```python
from build123d import *

# Parameters (mm, degrees)
SKETCH1_R           = 1.6
BOSS_EXTRUDE1_DEPTH = 9
FILLET1_R           = 10


with BuildPart() as part:
    # Sketch1 → Boss-Extrude1 (new body)
    with BuildSketch(Plane.XY):
        with BuildLine():
            Line((-3.813815801, 22.581093964), (4.789830745, 10.293813299))
            Line((4.789830745, 10.293813299), (2.332374612, 8.57308399))
            Line((2.332374612, 8.57308399), (-3.837793208, 17.384996862))
            ThreePointArc((-3.837793208, 17.384996862), (-10.92541976, 17.081695789), (-9.5, 24.031128874))
            Line((-9.5, 24.031128874), (-9.5, 60))
            Line((-9.5, 60), (-5.5, 60))
            Line((-5.5, 60), (-5.5, 24.031128874))
            ThreePointArc((-5.5, 24.031128874), (-4.565920417, 23.41191691), (-3.813815801, 22.581093964))
        make_face()
        with Locations((-7.5, 20)):
            Circle(SKETCH1_R, mode=Mode.SUBTRACT)
    extrude(amount=BOSS_EXTRUDE1_DEPTH)

    # Fillet1
    fillet1_edges = [part.edges().sort_by_distance(p)[0] for p in [
        (-3.837793208, 17.384996862, 4.5),
        (-9.5, 24.031128874, 4.5),
        (-5.5, 24.031128874, 4.5),
    ]]
    fillet(fillet1_edges, radius=FILLET1_R)


solid = part.part
```
Could you check a few things on this model? Use its own coordinates, in mm. A direction names the side the tool comes from. Round coordinates to 2 decimals unless told otherwise and drop trailing zeros. Order: outer loops, then holes, each group sorted by start corner. A loop starts at its lowest first (then second) coordinate and runs counter-clockwise, first axis right, second up. Notation, with made-up numbers: M 21,80 L 44,80 A30 ccw 44,107 Z; hole C 6.25,58 d4. An arc over 180 degrees is marked long. One line per question, with ' | ' between items. Start each with the question number.
(1) Suppose I cut it at A-A on y = 20. List the corners of the cut face in (x, z) for me, then the cut area to 3 significant figures.
(2) For P1, Ø5, axis at x = -6.5, z = 7.5, coming from the -Y side; P2, Ø2, axis at x = 3, z = 1, coming from the +Y side; P3, Ø4, axis at y = 46.5, z = 5, coming from the -X side, each with a flat end and sliding along its axis, tell me the tip position at first contact or that it passes through.
(3) Thinking about a two-plate mould opening in Y: for faces 1 (the face through (1.41, 9.89, 4.44)), 2 (the face through (-7, 33, 0)), 3 (the face through (-7.708, 21.586, 4.437)), which applies, +Y half, -Y half, draft (parallel to the pull), parting line (faces both ways), or undercut?
(4) Suppose I cut it at B-B on x = -0.5. List the corners of the cut face in (y, z) for me, then the cut area to 3 significant figures.
(5) Suppose I cut it at C-C on y = 53. List the corners of the cut face in (x, z) for me.
(6) Please list where these lines run through material, in increasing order: line 1 along Y through (x, z) = (-7.5, 2); line 2 along X through (y, z) = (33, 7.5); line 3 along Y through (x, z) = (-8.5, 4.5).
(7) For faces 4 (the face through (-5.5, 44, 4)), 5 (the face through (-9.5, 44, 4)), 6 (the face through (-11.46, 17.86, 4.44)), which set-ups out of +Z, -Z, +X, -X, +Y, -Y let a thin tool reach every point of the face, with its end or its side?
Geometry results:
1) outline: M -12,0 L -9.1,0 L -9.1,9 L -12,9 Z; M -5.9,0 L -2.01,0 L -2.01,9 L -5.9,9 Z | area: 61.1 mm²
2) P1: y = 14.78 | P2: y = 14.28 | P3: x = -9.5
3) face 1: -Y half | face 2: draft | face 3: undercut
4) outline: M 12.42,0 L 17.85,0 L 17.85,9 L 12.42,9 Z | area: 48.9 mm²
5) outline: M -9.5,0 L -5.5,0 L -5.5,9 L -9.5,9 Z
6) line 1: 15.5 to 18.4, 21.6 to 60 | line 2: -9.5 to -5.5 | line 3: 15.61 to 18.75, 21.25 to 60
7) face 4: +Z, -Z, +X, +Y | face 5: +Z, -Z, -X, +Y | face 6: +Z, -Z, -X
